For this review, take the finished solid that the model builds, in its own axes (mm). A direction names the side the tool comes from. Give positions to 0.01 mm unless a question says otherwise; leave off trailing zeros. Loops run counter-clockwise (first coordinate to the right, second up) from the corner with the lowest first, then second, coordinate; pieces in that order, holes last. Notation, with made-up numbers: (21.5, 31) -> (31.5, 31) arc R14 ccw to (31.5, 57) -> close; hole circle Ø5 at (-27, -31.5). An arc over 180 degrees is marked (long way). One line per question, with ' | ' between items. Start each with the question number.
(1) Wall thickness on probe 1 along X at (y, z) = (10, 13.5); probe 2 along Z at (x, y) = (40.5, 6.75); probe 3 along X at (y, z) = (14, 32.5): over which ranges is each line inside the solid? List them lowest first.
(2) Draft analysis for pull direction X (two halves, no side actions). For faces 1 (the flat face through (60, 10, 30)), 2 (the flat face through (0, 7, 30)), 3 (the flat face through (80, 7, 30)), state which applies: +X half, -X half, draft (parallel to the pull), parting line (faces both ways), or undercut.
(3) Consider section A-A (z = 38). Write out the cut boundary in (x, y).
(4) Consider section C-C (x = 49.5). Write out the cut boundary in (y, z), and give its area (3 significant figures).
(5) Tool access review of faces 4 (the flat face through (40, 2, 3)), 5 (the flat face through (40, 7, 0)), 6 (the flat face through (40, 10, 11)): name each direction out of +Z, -Z, +X, -X, +Y, -Y from which nothing blocks a thin tool from reaching the whole face with its end or side.
(6) Consider section B-B (y = 9.25). Write out the cut boundary in (x, z).
(7) Insertion check: P1, Ø1.5, axis at y = 11, z = 51.5, coming from the -X side; P2, Ø3, axis at x = 64.5, z = 47.5, coming from the -Y side; P3, Ø3, axis at x = 66, z = 12, coming from the -Y side. Each pin has a flat end and moves straight along its axis. Give the tip position at first contact, or say it passes through.
(8) Consider section D-D (y = 2.5). Write out the cut boundary in (x, z), and give its area (3 significant figures).
from build123d import *

# Parameters (mm, degrees)
BOSS_EXTRU_1_DEPTH      = 15
ENL_V_MAT_EXTRU_1_DEPTH = 5
ESQUISSE3_R             = 2.8
ENL_V_MAT_EXTRU_2_DEPTH = 8.1


with BuildPart() as part:
    # Esquisse1 → Boss.-Extru.1 (new body)
    with BuildSketch(Plane(origin=(0, 0, 0), x_dir=(1, 0, 0), z_dir=(0, 1, 0))):
        with BuildLine():
            Line((10, 0), (70, 0))
            ThreePointArc((70, 0), (77.071067812, -2.928932188), (80, -10))
            Line((80, -10), (80, -50))
            ThreePointArc((80, -50), (77.071067812, -57.071067812), (70, -60))
            Line((70, -60), (10, -60))
            ThreePointArc((10, -60), (2.928932188, -57.071067812), (0, -50))
            Line((0, -50), (0, -10))
            ThreePointArc((0, -10), (2.928932188, -2.928932188), (10, 0))
        make_face()
        with BuildLine():
            Line((58, -49), (22, -49))
            ThreePointArc((22, -49), (20.585786438, -48.414213562), (20, -47))
            Line((20, -47), (20, -13))
            ThreePointArc((20, -13), (20.585786438, -11.585786438), (22, -11))
            Line((22, -11), (58, -11))
            ThreePointArc((58, -11), (59.414213562, -11.585786438), (60, -13))
            Line((60, -13), (60, -47))
            ThreePointArc((60, -47), (59.414213562, -48.414213562), (58, -49))
        make_face(mode=Mode.SUBTRACT)
    extrude(amount=BOSS_EXTRU_1_DEPTH)

    # Esquisse2 → Enlèv. mat.-Extru.1 (cut)
    with BuildSketch(Plane.XZ):
        with BuildLine():
            Line((8, 57), (72, 57))
            ThreePointArc((72, 57), (75.535533906, 55.535533906), (77, 52))
            Line((77, 52), (77, 8))
            ThreePointArc((77, 8), (75.535533906, 4.464466094), (72, 3))
            Line((72, 3), (8, 3))
            ThreePointArc((8, 3), (4.464466094, 4.464466094), (3, 8))
            Line((3, 8), (3, 52))
            ThreePointArc((3, 52), (4.464466094, 55.535533906), (8, 57))
        make_face()
    extrude(amount=-ENL_V_MAT_EXTRU_1_DEPTH, mode=Mode.SUBTRACT)

    # Esquisse3 → Enlèv. mat.-Extru.2 (cut)
    with BuildSketch(Plane.XZ.offset(-5)):
        with Locations(Location((65, 13.5, 0), (0, 0, 270))):
            Circle(ESQUISSE3_R)
        with Locations(Location((65, 46.5, 0), (0, 0, 270))):
            Circle(ESQUISSE3_R)
        with Locations(Location((15, 13.5, 0), (0, 0, 270))):
            Circle(ESQUISSE3_R)
        with Locations(Location((15, 46.5, 0), (0, 0, 270))):
            Circle(ESQUISSE3_R)
    extrude(amount=-ENL_V_MAT_EXTRU_2_DEPTH, mode=Mode.SUBTRACT)


solid = part.part
A:
1) probe 1: x = 0 to 12.2, 17.8 to 20, 60 to 62.2, 67.8 to 80 | probe 2: z = 0 to 11, 49 to 60 | probe 3: x = 0 to 20, 60 to 80
2) face 1: undercut | face 2: -X half | face 3: +X half
3) outline: (0, 0) -> (3, 0) -> (3, 5) -> (20, 5) -> (20, 15) -> (0, 15) -> close; (60, 5) -> (77, 5) -> (77, 0) -> (80, 0) -> (80, 15) -> (60, 15) -> close
4) outline: (0, 0) -> (15, 0) -> (15, 11) -> (5, 11) -> (5, 3) -> (0, 3) -> close; (0, 57) -> (5, 57) -> (5, 49) -> (15, 49) -> (15, 60) -> (0, 60) -> close | area: 250 mm^2
5) face 4: -Y | face 5: -Z, +X, -X, +Y, -Y | face 6: +Y, -Y
6) outline: (0, 10) arc R10 ccw to (10, 0) -> (70, 0) arc R10 ccw to (80, 10) -> (80, 50) arc R10 ccw to (70, 60) -> (10, 60) arc R10 ccw to (0, 50) -> close; hole circle Ø5.6 at (15, 13.5); hole circle Ø5.6 at (15, 46.5); hole (20, 13) arc R2 ccw to (22, 11) -> (58, 11) arc R2 ccw to (60, 13) -> (60, 47) arc R2 ccw to (58, 49) -> (22, 49) arc R2 ccw to (20, 47) -> close; hole circle Ø5.6 at (65, 13.5); hole circle Ø5.6 at (65, 46.5)
7) P1: stops at x = 0.03 | P2: stops at y = 13.1 | P3: stops at y = 5
8) outline: (0, 10) arc R10 ccw to (10, 0) -> (70, 0) arc R10 ccw to (80, 10) -> (80, 50) arc R10 ccw to (70, 60) -> (10, 60) arc R10 ccw to (0, 50) -> close; hole (3, 8) arc R5 ccw to (8, 3) -> (72, 3) arc R5 ccw to (77, 8) -> (77, 52) arc R5 ccw to (72, 57) -> (8, 57) arc R5 ccw to (3, 52) -> close | area: 740 mm^2
